For this review, use the dimensioned drawing (mm, ordinates from the lowest corner) and the shaded views. A direction names the side the tool comes from. Give positions to 0.01 mm unless a question says otherwise; leave off trailing zeros. Loops run counter-clockwise (first coordinate to the right, second up) from the corner with the lowest first, then second, coordinate; pieces in that order, holes last. Notation, with made-up numbers: (-10.5, 37.25) - (-3.5, 37.25) arc R20 ccw to (-3.5, 73.25) - close; hole circle Ø2 at (26.5, 29). An arc over 180 degrees is marked (long way). Write each question's results on one line, items separated by ' | '.
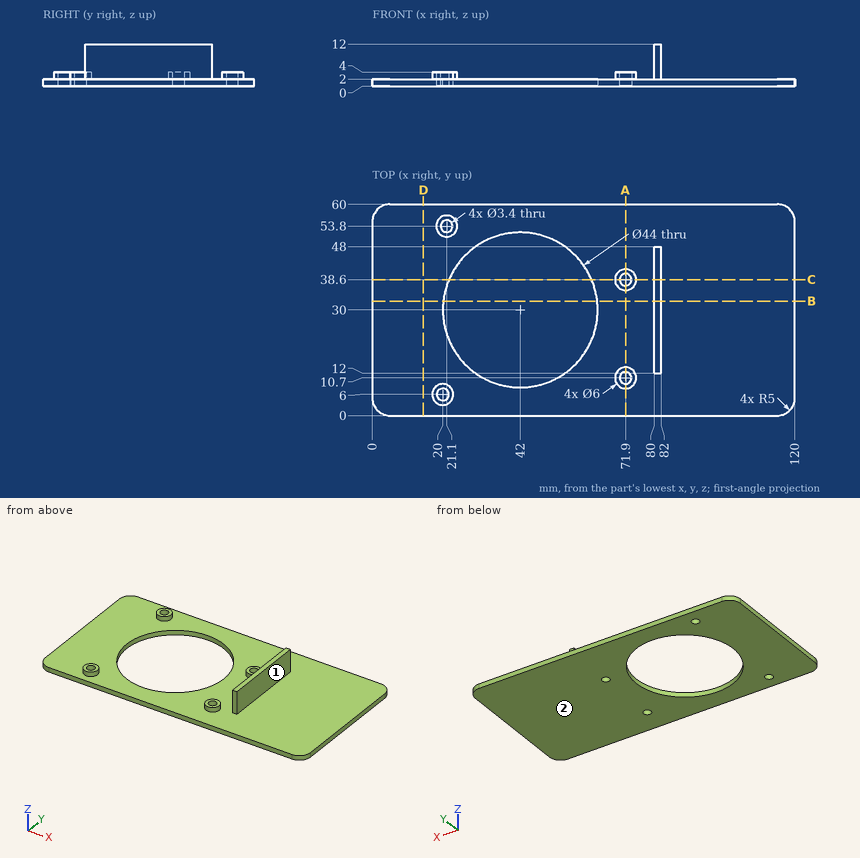
Item 1: We need section B-B on y = 32.5. Give the boundary of the cut face in (x, z), then the cut area to 3 significant figures.
Output values:
outline: (0, 0) - (20.14, 0) - (20.14, 2) - (0, 2) - close; (63.86, 0) - (120, 0) - (120, 2) - (82, 2) - (82, 12) - (80, 12) - (80, 2) - (63.86, 2) - close | area: 173 mm²
Item 2: We need section C-C on y = 38.6. Give the boundary of the cut face in (x, z).
Output values:
outline: (0, 0) - (21.75, 0) - (21.75, 2) - (0, 2) - close; (62.25, 0) - (70.2, 0) - (70.2, 4) - (68.9, 4) - (68.9, 2) - (62.25, 2) - close; (73.6, 0) - (120, 0) - (120, 2) - (82, 2) - (82, 12) - (80, 12) - (80, 2) - (74.9, 2) - (74.9, 4) - (73.6, 4) - close
Item 3: Clearance check with flat-ended pins moving along their axes: P1, Ø6, axis at y = 37.5, z = 6.5, coming from the +X side; P2, Ø1, axis at x = 81, z = 6.5, coming from the -Y side; P3, Ø3, axis at x = 20, y = 54, coming from the +Z side. State where each tip first meets the part, or that it passes through.
Output values:
P1: stops at x = 82 | P2: stops at y = 12 | P3: stops at z = 4
Item 4: Tool access review of the marked faces 1 and 2: name each direction out of +Z, -Z, +X, -X, +Y, -Y from which nothing blocks a thin tool from reaching the whole face with its end or side.
Output values:
face 1: +Z, +X, +Y, -Y | face 2: -Z, +X, -X, +Y, -Y
Item 5: We need section A-A on x = 71.9. Give the boundary of the cut face in (y, z), then the cut area to 3 significant figures.
Output values:
outline: (0, 0) - (9, 0) - (9, 4) - (7.7, 4) - (7.7, 2) - (0, 2) - close; (12.4, 0) - (36.9, 0) - (36.9, 4) - (35.6, 4) - (35.6, 2) - (13.7, 2) - (13.7, 4) - (12.4, 4) - close; (40.3, 0) - (60, 0) - (60, 2) - (41.6, 2) - (41.6, 4) - (40.3, 4) - close | area: 117 mm²
Item 6: Wall thickness on probe 1 along Y at (x, z) = (20, 3.1); probe 2 along Y at (x, z) = (71.9, 3.2); probe 3 along X at (y, z) = (29.5, 1.5): over which ranges is each line inside the solid? List them lowest first.
Output values:
probe 1: y = 3 to 4.3, 7.7 to 9, 51.01 to 52.5, 55.1 to 56.59 | probe 2: y = 7.7 to 9, 12.4 to 13.7, 35.6 to 36.9, 40.3 to 41.6 | probe 3: x = 0 to 20.01, 63.99 to 120
Item 7: We need section D-D on x = 14.5. Give the boundary of the cut face in (y, z), then the cut area to 3 significant figures.
Output values:
outline: (0, 0) - (60, 0) - (60, 2) - (0, 2) - close | area: 120 mm²
